from build123d import *

# Parameters (mm, degrees)
F0_W     = 105
F0_H     = 20
F1_DEPTH = 3
F2_R     = 6
F2_R_2   = 5
F3_DEPTH = 25
F5_W     = 10
F5_H     = 10
F6_DEPTH = 8.9
F4_W     = 10
F4_H     = 10
F7_DEPTH = 9
F8_R     = 2.50333
F8_R_2   = 2.524532
F9_DEPTH = 25


with BuildPart() as f1:
    # F0 (on Front) → F1 (new body)
    with BuildSketch(Plane.XZ):
        Rectangle(F0_W, F0_H)
    extrude(amount=F1_DEPTH)

    # F2 (on face) → F3 (cut)
    with BuildSketch(Plane.XZ.offset(3)):
        Circle(F2_R)
        with Locations((-41.33, 0)):
            Circle(F2_R_2)
        with Locations((41.33, 0)):
            Circle(F2_R_2)
    extrude(amount=-F3_DEPTH, mode=Mode.SUBTRACT)

    # F5 (on face) → F6 (join)
    with BuildSketch(Plane.XZ.offset(3)):
        with Locations((28, 0)):
            Rectangle(F5_W, F5_H)
    extrude(amount=F6_DEPTH)

    # F4 (on face) → F7 (join)
    with BuildSketch(Plane.XZ.offset(3)):
        with Locations((-11, 0)):
            Rectangle(F4_W, F4_H)
    extrude(amount=F7_DEPTH)

    # F8 (on face) → F9 (cut)
    with BuildSketch(Plane.XZ.offset(12)):
        with Locations((-9, 0)):
            Circle(F8_R)
        with Locations((26.3, 0)):
            Circle(F8_R_2)
    extrude(amount=-F9_DEPTH, mode=Mode.SUBTRACT)


solid = f1.part
Geometry check sheet. Reference: the model listing, model coordinates, mm. A direction names the side the tool comes from. Round coordinates to 2 decimals unless told otherwise and drop trailing zeros. Order: outer loops, then holes, each group sorted by start corner. A loop starts at its lowest first (then second) coordinate and runs counter-clockwise, first axis right, second up. Notation, with made-up numbers: (24, -3) - (58, -3) arc R7 ccw to (58, 4) - close; hole circle Ø7 at (24.5, -25). An arc over 180 degrees is marked (long way). One line per question, with ' | ' between items. Start each with the question number.
(1) Thickness scan on L1, parallel to Z at x = 26.3, y = -9.25; L2, parallel to Z at x = 41.33, y = -2.3; L3, parallel to X at y = -2.5, z = -1.75. Record the ranges inside material, lowest first. Write a range as [from, to].
(2) Depth check by flat-ended pin: pin 1 Ø7 at (x, y) = (29.5, -7) entering from -Z; pin 2 Ø3 at (x, z) = (29, -1.5) entering from -Y; pin 3 Ø1.5 at (x, z) = (-35, -0.5) entering from -Y. Enter the tip coordinate at first touch or a pass-through.
(3) Access from +Z, -Z, +X, -X, +Y, -Y to the whole of each face (thin tool, end or side, straight path). Record for faces 1 (the flat face through (-11, -7, 5)), 2 (the flat face through (28, -7, -5)), 3 (the flat face through (-6, -7, 0)).
(4) Sectioned sample at A-A on y = -8. Record the cut outline in (x, z).
(5) Sectioned sample at D-D on x = 26.3. Record the cut outline in (y, z), and give its area (3 significant figures).
(6) Release check for a two-part mould opening along Z. For faces 4 (the cylindrical face through (-6.61, -6.08, 0.75)), 5 (the flat face through (-1, -1, 10)), 6 (the flat face through (-1, -3, 7)) record: released by +Z, released by -Z, zero draft, split by the parting line, or undercut.
(7) Sectioned sample at C-C on y = -2. Record the cut outline in (x, z).
(8) Sectioned sample at B-B on x = -41.33. Record the cut outline in (y, z).
Conclusion:
1) L1: z = [-5, -2.52], [2.52, 5] | L2: z = [-10, -5], [5, 10] | L3: x = [-52.5, -46.01], [-36.65, -10.79], [-7.21, -5.74], [5.74, 24.48], [28.12, 36.65], [46.01, 52.5]
2) pin 1: stops at z = -5 | pin 2: stops at y = -11.9 | pin 3: stops at y = -3
3) face 1: +Z, +X, -X, -Y | face 2: -Z, +X, -X, -Y | face 3: +Z, -Z, -Y
4) outline: (-16, -5) - (-6, -5) - (-6, 5) - (-16, 5) - close; (23, -5) - (33, -5) - (33, 5) - (23, 5) - close; hole circle Ø5.01 at (-9, 0); hole circle Ø5.05 at (26.3, 0)
5) outline: (-11.9, -5) - (-3, -5) - (-3, -10) - (0, -10) - (0, -2.52) - (-11.9, -2.52) - close; (-11.9, 2.52) - (0, 2.52) - (0, 10) - (-3, 10) - (-3, 5) - (-11.9, 5) - close | area: 88.9 mm2
6) face 4: undercut | face 5: released by +Z | face 6: zero draft
7) outline: (-52.5, -10) - (52.5, -10) - (52.5, 10) - (-52.5, 10) - close; hole circle Ø10 at (-41.33, 0); hole circle Ø5.01 at (-9, 0); hole circle Ø12 at (0, 0); hole circle Ø5.05 at (26.3, 0); hole circle Ø10 at (41.33, 0)
8) outline: (-3, -10) - (0, -10) - (0, -5) - (-3, -5) - close; (-3, 5) - (0, 5) - (0, 10) - (-3, 10) - close
